Study the drawing (mm; zero at the part's minimum x, y, z) and answer. A direction names the side the tool comes from. Round coordinates to 2 decimals unless told otherwise and drop trailing zeros. Loops run counter-clockwise (first coordinate to the right, second up) from the corner with the lowest first, then second, coordinate; pieces in that order, holes last. Notation, with made-up numbers: M -33.75,80 L -18.75,80 A19 ccw -18.75,114 Z; hole C 75.5,67 d8. An arc over 180 degrees is marked long. Put each result on its own line as item: value. Start each with the question number.
(1) Flat-ended cylindrical pins translate along their axes: P1, Ø3, axis at x = 6.5, y = 1.5, coming from the +Z side; P2, Ø2, axis at y = 2, z = 9, coming from the +X side; P3, Ø0.9, axis at x = 18, y = 3.5, coming from the -Z side. Find the tip coordinate at first contact, or state that the pin passes through.
(2) Straight lines are drawn through the part: line 1 (Y direction, x = 9.5, z = 21); line 2 (X direction, y = 0.6, z = 32.5) (1 decimal). For each, find the intervals that lie inside material, in ascending order.
(3) Section C-C, the plane y = 2.5 is taken. Determine the outline of the cut face in (x, z).
(4) Which of the six approach directions +Z, -Z, +X, -X, +Y, -Y give full straight-line access (tool end or side, diameter ignored) to the marked faces 1 and 2?
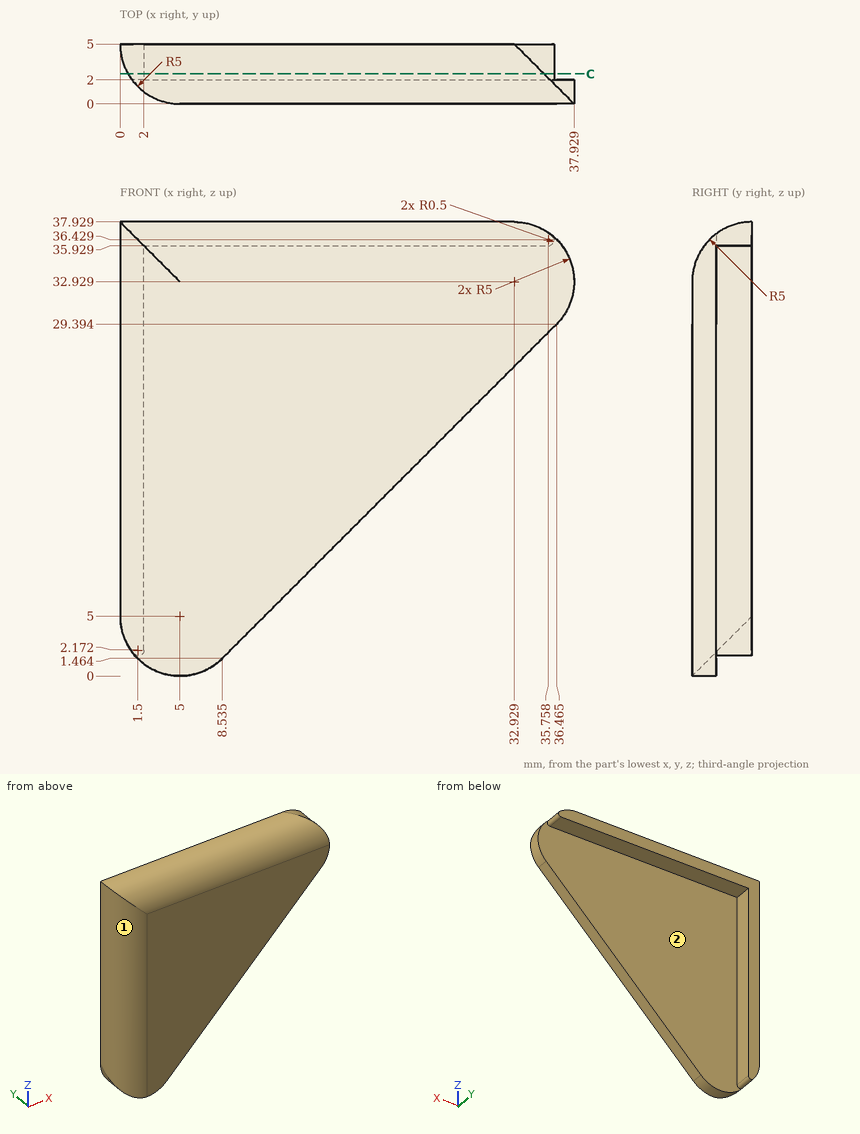
Recorded:
1. P1: stops at z = 37.51
1. P2: stops at x = 17.07
1. P3: stops at z = 35.93
2. line 1: y = 0 to 2
2. line 2: x = 2.6 to 37.9
3. outline: M 0.67,2.5 A5 ccw 1.11,1.86 A0.5 ccw 2,2.17 L 2,35.93 L 35.76,35.93 A0.5 ccw 36.07,36.82 A5 ccw 35.43,37.26 L 0.67,37.26 Z
4. face 1: +Z, -Z, -X, -Y
4. face 2: -Z, +X, +Y
